Source: three-view drawing plus pictorial views. Frame: mm from the lowest corner of the part. Give positions to 0.01 mm unless a question says otherwise; leave off trailing zeros. Loops run counter-clockwise (first coordinate to the right, second up) from the corner with the lowest first, then second, coordinate; pieces in that order, holes last.
1. Section A-A, the plane y = 43. Output: boundary loops of the cut face in (x, z).
2. Section D-D, the plane y = 17.5. Output: boundary loops of the cut face in (x, z), then the cut area to 3 significant figures.
3. Material intervals for line 1 along Y through (x, z) = (91, 3.35); line 2 along X through (y, z) = (37.5, 4.5); line 3 along Y through (x, z) = (51.5, 4.6), sorted ascending.
4. Section C-C, the plane z = 1.55. Output: boundary loops of the cut face in (x, y), then the cut area to 3 significant figures.
5. Section B-B, the plane x = 75. Output: boundary loops of the cut face in (y, z).
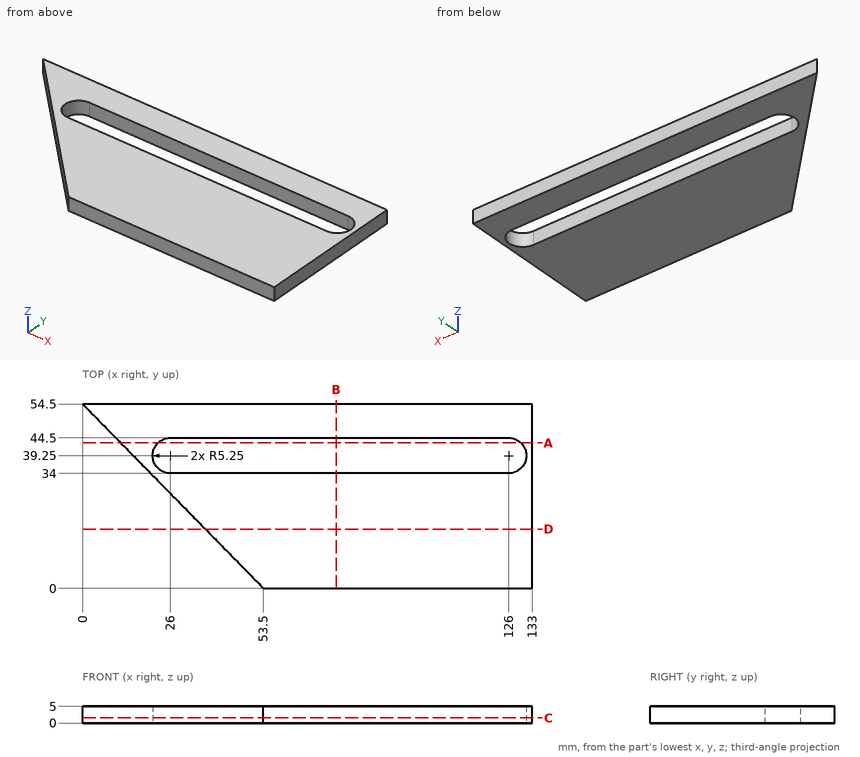
Answers below:
1. outline: (11.29, 0) - (22.33, 0) - (22.33, 5) - (11.29, 5) - close; (129.67, 0) - (133, 0) - (133, 5) - (129.67, 5) - close
2. outline: (36.32, 0) - (133, 0) - (133, 5) - (36.32, 5) - close
2. area: 483 mm2
3. line 1: y = 0 to 34, 44.5 to 54.5
3. line 2: x = 16.69 to 21.05, 130.95 to 133
3. line 3: y = 2.04 to 34, 44.5 to 54.5
4. outline: (0, 54.5) - (53.5, 0) - (133, 0) - (133, 54.5) - close; hole (26, 34) - (126, 34) arc R5.25 ccw to (126, 44.5) - (26, 44.5) arc R5.25 ccw to start
4. area: 4,650 mm2
5. outline: (0, 0) - (34, 0) - (34, 5) - (0, 5) - close; (44.5, 0) - (54.5, 0) - (54.5, 5) - (44.5, 5) - close
